Autodesk Inventor part; units mm, degrees
ref_plane "YZ Plane" through (0, 0, 0) normal (1, 0, 0) x (0, 1, 0)
ref_plane "XZ Plane" through (0, 0, 0) normal (0, 1, 0) x (-1, 0, 0)
ref_plane "XY Plane" through (0, 0, 0) normal (0, 0, 1) x (1, 0, 0)
sketch "Sketch1" plane through (0, 0, 0) normal (0, 0, 1) x (1, 0, 0)
  circle A0 centre (0, 0) radius 30.734
  line L0 (-56.515, -58.42) -> (56.515, -58.42)
  line L1 (56.515, -58.42) -> (56.515, 335.28)
  line L2 (56.515, 335.28) -> (-13.335, 335.28)
  line L3 (-13.335, 335.28) -> (-56.515, -58.42)
  dimension "d0" = 61.468
  dimension "d1" = 393.7
  dimension "d2" = 113.03
  dimension "d3" = 69.85
  dimension "d4" = 58.42
  dimension "d5" = 56.515
extrude "Extrusion1" add sketch "Sketch1" against normal blind 54.3243
fillet "Fillet1" radius 30.48 2 edges at (56.515, 335.28, -27.1621) (-13.335, 335.28, -27.1621)
sketch "Sketch2" plane through (-56.515, -58.42, 0) normal (0, -1, 0) x (1, 0, 0)
  line L0 (113.03, 0) -> (113.03, -54.3243)
  line L1 (113.03, -27.1621) -> (0, -27.1621)
  line L2 (0, 0) -> (0, -54.3243)
  line L3 (56.515, -27.1621) -> (56.515, -44.3071)
  circle A0 centre (87.63, -27.1621) radius 25.4
  circle A1 centre (25.4, -27.1621) radius 25.4
  point P0 (56.515, 0)
  dimension "d10" = 50.8
  dimension "d9" = 50.8
  dimension "d11" = 113.03
extrude "Extrusion2" add sketch "Sketch2" along normal blind 71.12
sketch "Sketch3" plane through (0, 0, 0) normal (0, 0, 1) x (1, 0, 0)
  circle A0 centre (0, 0) radius 42.7153
extrude "Extrusion3" add sketch "Sketch3" against normal blind 33.02
sketch "Sketch4" plane through (0, 0, -54.3243) normal (0, 0, -1) x (-1, 0, 0)
  line L0 (-26.035, 335.28) -> (-13.9848, 335.28)
  line L1 (-20.0099, 335.28) -> (-20.0099, 292.1)
  circle A0 centre (-20.0099, 292.1) radius 18.415
  point P0 (0, 0)
  dimension "d17" = 36.83
  dimension "d20" = 292.1
extrude "Extrusion4" add sketch "Sketch4" against normal blind 83.82
equation "\"d10\" = d9"
properties part number "Forearm"
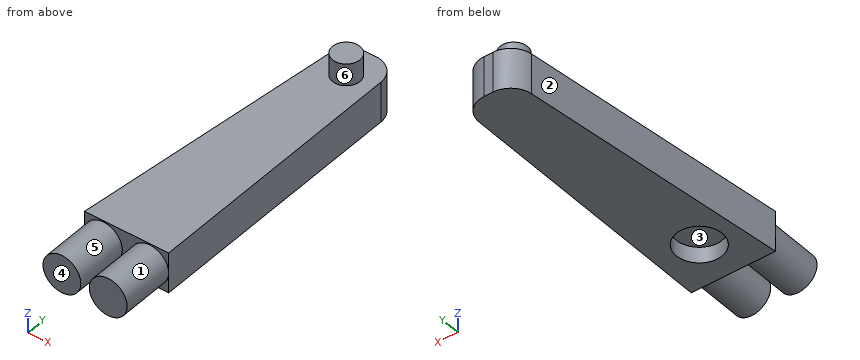
Verification items for the finished model (mm, model axes). Face numbers are marked on the shaded views. A direction names the side the tool comes from. Give positions to 0.01 mm unless a question says otherwise; leave off trailing zeros. Order: outer loops, then holes, each group sorted by start corner. A loop starts at its lowest first (then second) coordinate and runs counter-clockwise, first axis right, second up. Notation, with made-up numbers: M 81.25,-24 L 121.25,-24 A20 ccw 121.25,15 Z; hole C 26,46.25 d9. An arc over 180 degrees is marked long. Return JSON: item names as keys, results as strings. Group by question number.
1) Section check C-C on z = 14.5. Record the cut outline in (x, y) (3 decimals), and give its area (3 significant figures).
2) Section check B-B on x = 48. Record the cut outline in (y, z), and give its area (3 significant figures).
3) Section check A-A on y = 292.1. Record the cut outline in (x, z) (3 decimals).
4) Scan lines: line 1 (Z direction, x = -0.5, y = 264); line 2 (Y direction, x = 15, z = -36.5); line 3 (Y direction, x = 0, z = -39). Record each from-to range of solid material in increasing order.
5) Section check D-D on x = 18. Record the cut outline in (y, z), and give its area (3 significant figures).
6) Go/stop test with flat-tipped pins: pin 1 Ø5 at (x, z) = (41.5, -22.5) entering from +Y; pin 2 Ø6 at (x, y) = (-22, 22.5) entering from +Z; pin 3 Ø4 at (x, z) = (-27.5, 1) entering from -Y. Record where each tip stops, or that it passes through.
7) Mould release check, pull along X, two halves, no side actions. Record for the marked faces 4, 5 and 6: pulls with the +X half, pulls with the -X half, needs draft (parallel to the pull), parting line crosses it, or undercut.
8) Access from +Z, -Z, +X, -X, +Y, -Y to the whole of each face (thin tool, end or side, straight path). Record for the marked faces 1, 2 and 3.
Answer block:
{
 "1": {"outline": "C 20.01,292.1 d36.83", "area": "1,070 mm^2"},
 "2": {"outline": "M -129.54,-46.14 L -58.42,-46.14 L -58.42,-54.32 L 325.93,-54.32 L 325.93,0 L -58.42,0 L -58.42,-8.19 L -129.54,-8.19 Z", "area": "23,600 mm^2"},
 "3": {"outline": "M -18.071,-54.324 L 56.515,-54.324 L 56.515,0 L 38.425,0 L 38.425,29.496 L 1.595,29.496 L 1.595,0 L -18.071,0 Z"},
 "4": {"line 1": "z = -54.32 to 0", "line 2": "y = -129.54 to -26.82, 26.82 to 335.28", "line 3": "y = -58.42 to -30.73, 30.73 to 331.88"},
 "5": {"outline": "M -129.54,-48.91 L -58.42,-48.91 L -58.42,-54.32 L -24.91,-54.32 L -24.91,-33.02 L 24.91,-33.02 L 24.91,-54.32 L 335.28,-54.32 L 335.28,0 L 310.4,0 L 310.4,29.5 L 273.8,29.5 L 273.8,0 L -58.42,0 L -58.42,-5.41 L -129.54,-5.41 Z", "area": "24,500 mm^2"},
 "6": {"pin 1": "stops at y = 332.39", "pin 2": "stops at z = 0", "pin 3": "stops at y = -58.42"},
 "7": {"face 4": "needs draft", "face 5": "undercut", "face 6": "parting line crosses it"},
 "8": {"face 1": "-Y", "face 2": "+Z, -Z, -X, +Y", "face 3": "-Z"}
}
